from build123d import *

# Parameters (mm, degrees)
BOSS_EXTRUDE1_DEPTH            = 3
SKETCH2_R                      = 1.95
BOSS_EXTRUDE2_DEPTH            = 3
M3_CLEARANCE_HOLE1_D           = 3.4
M3_CLEARANCE_HOLE1_CSINK_D     = 3.45
M3_CLEARANCE_HOLE1_CSINK_ANGLE = 90


with BuildPart() as part:
    # Sketch1 → Boss-Extrude1 (new body)
    with BuildSketch(Plane.XY):
        with BuildLine():
            Line((-11.9, 0), (-11.9, -22.34))
            Line((-11.9, -22.34), (11.9, -22.34))
            Line((11.9, -22.34), (11.9, 0))
            ThreePointArc((11.9, 0), (0, 11.9), (-11.9, 0))
        make_face()
    extrude(amount=BOSS_EXTRUDE1_DEPTH)

    # Sketch2 → Boss-Extrude2 (add)
    with BuildSketch(Plane(origin=(0, 0, 0), x_dir=(-1, 0, 0), z_dir=(0, 0, -1))):
        with Locations(Location((0, 6, 0), (0, 0, 180))):
            Circle(SKETCH2_R)
        with Locations(Location((6, 0, 0), (0, 0, 180))):
            Circle(SKETCH2_R)
        with Locations(Location((0, -6, 0), (0, 0, 180))):
            Circle(SKETCH2_R)
        with Locations(Location((-6, 0, 0), (0, 0, 180))):
            Circle(SKETCH2_R)
    extrude(amount=BOSS_EXTRUDE2_DEPTH)

    # M3 Clearance Hole1 (through all)
    with Locations(Plane(origin=(-5.9, -15.34, 3), x_dir=(1, 0, 0), z_dir=(0, 0, 1))):
        with Locations((0, 0), (11.8, 0)):
            CounterSinkHole(M3_CLEARANCE_HOLE1_D / 2, M3_CLEARANCE_HOLE1_CSINK_D / 2, counter_sink_angle=M3_CLEARANCE_HOLE1_CSINK_ANGLE)


solid = part.part
Verification items for the finished model (mm, model axes). A direction names the side the tool comes from. Coordinates: 2 decimals unless noted, no trailing zeros. Write each loop counter-clockwise with the first axis right and the second up, starting at its lowest first coordinate (ties: lowest second). Pieces come first, ordered by that corner, then holes. Notation, with made-up numbers: (4.5, 24.5) -> (45.5, 24.5) arc R30 cw to (45.5, 59.5) -> close; hole circle Ø1 at (-18.75, -13). An arc over 180 degrees is marked (long way). One line per item, written item: value. Start each with the question number.
Q1. Mould release check, pull along X, two halves, no side actions. Record for faces 3 (the cylindrical face through (-7.52, -14.83, 1.47)), 4 (the flat face through (0, -6, -3)), 5 (the cylindrical face through (-0.423, 7.904, -1.479)): pulls with the +X half, pulls with the -X half, needs draft (parallel to the pull), parting line crosses it, or undercut.
Q2. Cross-section at B-B on z = -2.3. Enter the section's corners in (x, y).
Q3. Cross-section at A-A on y = -15.34. Enter the section's corners in (x, z) (3 decimals), and give its area (3 significant figures).
Q4. Thickness scan on L1, parallel to X at y = -15.34, z = 2.05; L2, parallel to Z at x = 3.25, y = 0; L3, parallel to Y at x = -5.9, z = 1. Record the ranges inside material, lowest first. Write a range as from..to.
Q5. Cross-section at C-C on x = 5.9. Enter the section's corners in (y, z) (3 decimals).
Q6. Go/stop test with flat-tipped pins: P1, Ø5, axis at x = -3.5, y = -18, coming from the -Z side; P2, Ø2, axis at x = 3, z = 1, coming from the +Y side; P3, Ø2.5, axis at x = 5.9, y = -15.34, coming from the +Z side. Record where each tip stops, or that it passes through.
Q7. Access from +Z, -Z, +X, -X, +Y, -Y to the whole of each face (thin tool, end or side, straight path). Record for faces 1 (the flat face through (6, 0, -3)), 2 (the cylindrical face through (4.052, -0.086, -1.479)).
Q8. Cross-section at D-D on y = -6. Enter the section's corners in (x, z), and give its area (3 significant figures).
Checked values:
1. face 3: undercut
1. face 4: needs draft
1. face 5: parting line crosses it
2. outline: circle Ø3.9 at (-6, 0); circle Ø3.9 at (0, -6); circle Ø3.9 at (0, 6); circle Ø3.9 at (6, 0)
3. outline: (-11.9, 0) -> (-7.6, 0) -> (-7.6, 2.975) -> (-7.625, 3) -> (-11.9, 3) -> close; (-4.2, 0) -> (4.2, 0) -> (4.2, 2.975) -> (4.175, 3) -> (-4.175, 3) -> (-4.2, 2.975) -> close; (7.6, 0) -> (11.9, 0) -> (11.9, 3) -> (7.625, 3) -> (7.6, 2.975) -> close
3. area: 51.0 mm²
4. L1: x = -11.9..-7.6, -4.2..4.2, 7.6..11.9
4. L2: z = 0..3
4. L3: y = -22.34..-17.04, -13.64..10.33
5. outline: (-22.34, 0) -> (-17.04, 0) -> (-17.04, 2.975) -> (-17.065, 3) -> (-22.34, 3) -> close; (-13.64, 0) -> (-1.947, 0) -> (-1.947, -3) -> (1.947, -3) -> (1.947, 0) -> (10.334, 0) -> (10.334, 3) -> (-13.615, 3) -> (-13.64, 2.975) -> close
6. P1: stops at z = 0
6. P2: stops at y = 11.73
6. P3: passes through
7. face 1: -Z, +X, -X, +Y, -Y
7. face 2: -Z
8. outline: (-11.9, 0) -> (-1.95, 0) -> (-1.95, -3) -> (1.95, -3) -> (1.95, 0) -> (11.9, 0) -> (11.9, 3) -> (-11.9, 3) -> close
8. area: 83.1 mm²
